Can you work these out from the model? Positions are in its coordinate system, mm. Face numbers are marked on the shaded views. Round coordinates to 2 decimals unless told otherwise and drop trailing zeros. Order: outer loops, then holes, each group sorted by start corner. A loop starts at its lowest first (then second) coordinate and runs counter-clockwise, first axis right, second up.
Q1. Will these pins go through, and if not, where does the flat tip stop? P1, Ø2, axis at y = -2, z = 59, coming from the +X side (3 decimals); P2, Ø10, axis at x = 7.5, z = 47, coming from the +Y side; P3, Ø10, axis at x = 7.5, z = 34.5, coming from the +Y side (3 decimals); P4, Ø4, axis at x = -1, z = 16, coming from the +Y side.
Q2. If we section it at A-A (x = 1.5): Please give me the cut outline in (y, z).
Q3. If we section it at C-C (z = 14.5): Please give me the cut outline in (x, y), plus the area to 3 significant figures.
Q4. We'd pull the mould along Y, two halves only. Please class the marked faces 1 and 2: pulls with the +Y half, pulls with the -Y half, needs draft (parallel to the pull), parting line crosses it, or undercut.
Q5. If we section it at B-B (y = 0): Please give me the cut outline in (x, z), plus the area to 3 significant figures.
Q6. If I drill on line 1 (X direction, y = 0, z = 41.5); line 2 (Y direction, x = 0, z = 67); line 3 (X direction, y = -16, z = 85), over which ranges is the centre line in solid material (lowest first)?
Q7. If we section it at D-D (z = 90.5): Please give me the cut outline in (x, y).
from build123d import *

# Parameters (mm, degrees)
SKETCH1_R               = 20
BOSS_EXTRUDE1_DEPTH     = 100
CUT_EXTRUDE1_DEPTH      = 104.923048454
CUT_EXTRUDE1_DEPTH_BACK = 104.923048454
SHELL1_OUTLINE_R        = 19.5
SHELL1_DEPTH            = 99.0625001


# Read off the part's stored shape, not the designer's step: Shell1
with BuildPart() as part:
    # Sketch1 → Boss-Extrude1 (new body)
    with BuildSketch(Plane.XY):
        Circle(SKETCH1_R)
    extrude(amount=BOSS_EXTRUDE1_DEPTH)

    # Sketch2 → Cut-Extrude1 (cut, two sides: drawn at the far end of the back side and taken through both)
    with BuildSketch(Plane(origin=(0, 0, 0), x_dir=(0, 0, -1), z_dir=(1, 0, 0)).offset(-CUT_EXTRUDE1_DEPTH_BACK)):
        Polygon((-100, -20), (-25, 20), (-100, 20), align=None)
    extrude(amount=CUT_EXTRUDE1_DEPTH + CUT_EXTRUDE1_DEPTH_BACK, mode=Mode.SUBTRACT)

    # Shell1 outline → Shell1 (cut)
    with BuildSketch(Plane.XY):
        Circle(SHELL1_OUTLINE_R)
    extrude(amount=SHELL1_DEPTH, mode=Mode.SUBTRACT)


solid = part.part
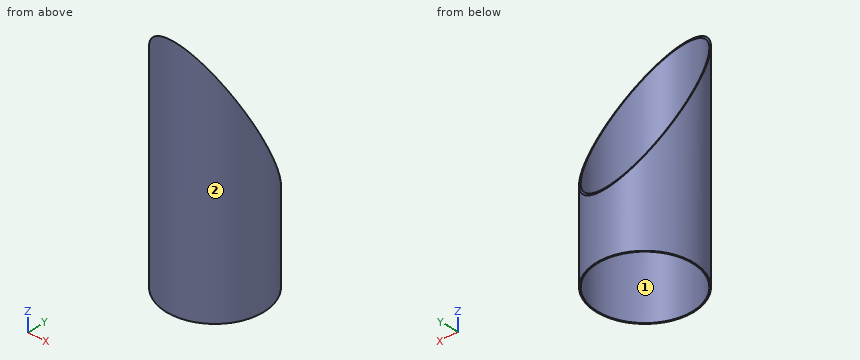
Solution:
1. P1: stops at x = 19.975
1. P2: stops at y = -14.97
1. P3: stops at y = 17.545
1. P4: stops at y = 20
2. outline: (-19.94, 0) - (-19.44, 0) - (-19.44, 98.95) - (-19.94, 99.89) - close; (19.44, 0) - (19.94, 0) - (19.94, 25.11) - (19.44, 26.05) - close
3. outline: circle Ø40 at (0, 0); hole circle Ø39 at (0, 0)
3. area: 62.0 mm2
4. face 1: undercut
4. face 2: parting line crosses it
5. outline: (-20, 0) - (-19.5, 0) - (-19.5, 62.5) - (-20, 62.5) - close; (19.5, 0) - (20, 0) - (20, 62.5) - (19.5, 62.5) - close
5. area: 62.5 mm2
6. line 1: x = -20 to -19.5, 19.5 to 20
6. line 2: y = -20 to -19.5
6. line 3: x = -12 to -11.15, 11.15 to 12
7. outline: (-13.3, -14.93) arc R20 ccw to (13.3, -14.93) - (12.54, -14.93) arc R19.5 cw to (-12.54, -14.93) - close
